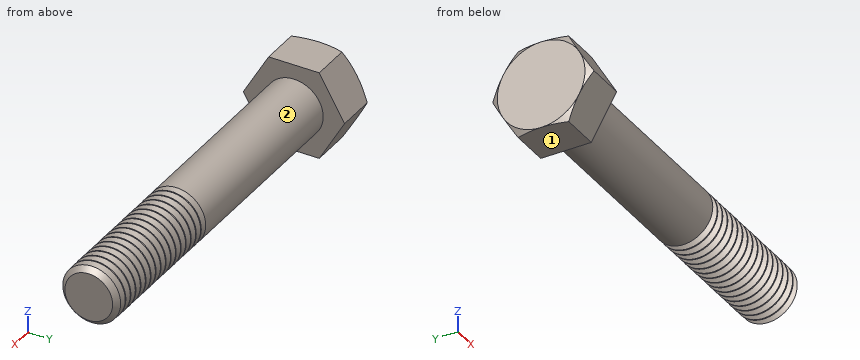
```python
from build123d import *

# Parameters (mm, degrees)
BASEHEAD_DEPTH  = 9.2456
THDSCHPAT_COUNT = 17
THDSCHPAT_PITCH = 1.867647059


with BuildPart() as part:
    # Sketch1 → BaseHead (new body)
    with BuildSketch(Plane(origin=(0, 0, 0), x_dir=(0, 0, -1), z_dir=(1, 0, 0))):
        Polygon((9.525, 5.499261314), (9.525, -5.499261314), (0, -10.998522628), (-9.525, -5.499261314), (-9.525, 5.499261314), (0, 10.998522628), align=None)
    extrude(amount=BASEHEAD_DEPTH)

    # BodySke → BaseBody (revolve)
    with BuildSketch(Plane.XY):
        Polygon((0, 0), (85.4456, 0), (85.4456, 5.18668), (84.28228, 6.35), (0, 6.35), align=None)
    revolve(axis=Axis((0, 0, 0), (1, 0, 0)))

    # Sketch3 → HeadChamfer (revolve, cut)
    with BuildSketch(Plane.XY):
        Polygon((0, 9.525), (4.516912895, 17.348522628), (4.516912895, 23.698522628), (-12.7, 23.698522628), (-12.7, 9.525), align=None)
    revolve(axis=Axis((0, 0, 0), (1, 0, 0)), mode=Mode.SUBTRACT)

    # ThdSchSke → ThreadSchematic (revolve, cut)
    with BuildSketch(Plane.XY):
        Polygon((53.6956, -5.18668), (52.881034567, -6.35), (52.881034567, -7.9375), (54.510165433, -7.9375), (54.510165433, -6.35), align=None)
    threadschematic = revolve(axis=Axis((-3.175, 0, 0), (1, 0, 0)), mode=Mode.SUBTRACT)

    # ThdSchPat: ThreadSchematic ×17
    with Locations(*[(i * THDSCHPAT_PITCH, 0, 0) for i in range(1, THDSCHPAT_COUNT)]):
        add(threadschematic, mode=Mode.SUBTRACT)


solid = part.part
```
Verification items for the finished model (mm, model axes). Face numbers are marked on the shaded views. A direction names the side the tool comes from. Give positions to 0.01 mm unless a question says otherwise; leave off trailing zeros. Loops run counter-clockwise (first coordinate to the right, second up) from the corner with the lowest first, then second, coordinate; pieces in that order, holes last. Notation, with made-up numbers: M 4,69.5 L 29,69.5 A8 ccw 29,73.5 Z; hole C -2.5,39.25 d5. An arc over 180 degrees is marked long. One line per question, with ' | ' between items.
Item 1: Depth check by flat-ended pin: P1, Ø3, axis at x = 15, y = 6, coming from the -Z side; P2, Ø1, axis at x = 19.5, z = 6, coming from the -Y side; P3, Ø1, axis at x = 23, y = 8, coming from the -Z side; P4, Ø3, axis at y = 7.5, z = 4, coming from the +X side. Enter the tip coordinate at first touch or a pass-through.
Completed:
P1: stops at z = -4.48 | P2: stops at y = -3.17 | P3: passes through | P4: stops at x = 9.25
Item 2: Tool access check on the marked faces 1 and 2. Record the directions out of +Z, -Z, +X, -X, +Y, -Y that give a thin tool (end or side, any length) a straight path to the whole face; none if there is none.
Completed:
face 1: -Z, +X, -X, +Y, -Y | face 2: +X
Item 3: Thickness scan on line 1 (X direction, y = 1.75, z = -6.75); line 2 (Y direction, x = 13.5, z = -0.25). Record the ranges inside material, lowest first. Write a range as [from, to].
Completed:
line 1: x = [0, 9.25] | line 2: y = [-6.35, 6.35]
Item 4: Section check A-A, the plane x = 20.5. Record the cut outline in (y, z), plus the area to 3 significant figures.
Completed:
outline: C 0,0 d12.7 | area: 127 mm^2
